```python
from build123d import *

# Parameters (mm, degrees)
SKETCH1_W           = 152.4
SKETCH1_H           = 101.6
BOSS_EXTRUDE1_DEPTH = 53.34
CUT_EXTRUDE1_START  = -12.7
SKETCH2_R           = 6.35
CUT_EXTRUDE1_DEPTH  = 127
FILLET2_R           = 2.54


with BuildPart() as part:
    # Sketch1 → Boss-Extrude1 (new body)
    with BuildSketch(Plane(origin=(0, 0, 0), x_dir=(1, 0, 0), z_dir=(0, 1, 0))):
        Rectangle(SKETCH1_W, SKETCH1_H)
    extrude(amount=-BOSS_EXTRUDE1_DEPTH)

    # Sketch2 → Cut-Extrude1 (cut)
    with BuildSketch(Plane(origin=(76.2, 0, 0), x_dir=(0, 0, -1), z_dir=(1, 0, 0)).offset(CUT_EXTRUDE1_START)):
        Circle(SKETCH2_R)
    extrude(amount=-CUT_EXTRUDE1_DEPTH, mode=Mode.SUBTRACT)

    # Fillet2
    fillet2_edges = [part.edges().sort_by_distance(p)[0] for p in [
        (63.5, -6.35, 0),
        (-63.5, -6.35, 0),
    ]]
    fillet(fillet2_edges, radius=FILLET2_R)


solid = part.part
```
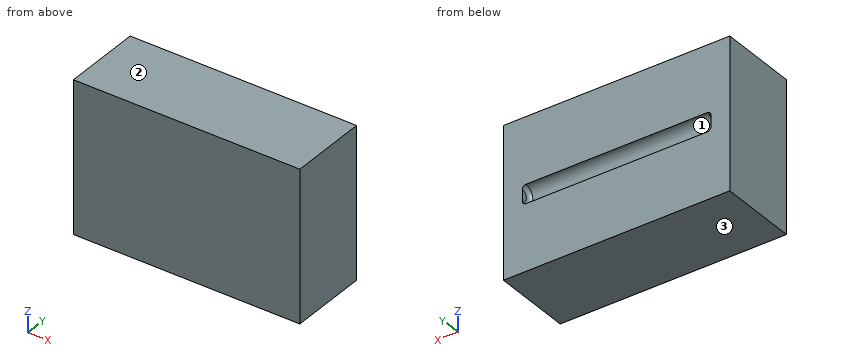
Read the model definition and answer for the solid it produces. Units are mm, in the model's axes. Face numbers are marked on the shaded views. Give positions to 0.01 mm unless a question says otherwise; leave off trailing zeros. Order: outer loops, then holes, each group sorted by start corner. A loop starts at its lowest first (then second) coordinate and runs counter-clockwise, first axis right, second up. Notation, with made-up numbers: (-4, -10.75) -> (10, -10.75) arc R23 ccw to (10, 12.25) -> close; hole circle Ø11 at (68.25, 71.25). An arc over 180 degrees is marked (long way). One line per item, written item: value. Start each with the question number.
(1) The part is cut by section A-A (z = 0). Determine the outline of the cut face in (x, y), and give its area (3 significant figures).
(2) Straight lines are drawn through the part: L1, parallel to Z at x = 60, y = -3; L2, parallel to Y at x = -59.5, z = -5. For each, find the intervals that lie inside material, in ascending order.
(3) For a pull along Z with two mould halves and no side action, classify the marked faces 1, 2 and 3 as released by +Z, released by -Z, zero draft, split by the parting line, or undercut.
Taken from the geometry:
1. outline: (-76.2, -53.34) -> (76.2, -53.34) -> (76.2, 0) -> (63.5, 0) -> (63.5, -3.81) arc R2.54 cw to (60.96, -6.35) -> (-60.96, -6.35) arc R2.54 cw to (-63.5, -3.81) -> (-63.5, 0) -> (-76.2, 0) -> close
1. area: 7,330 mm^2
2. L1: -50.8 to -5.6, 5.6 to 50.8
2. L2: -53.34 to -3.91
3. face 1: undercut
3. face 2: released by +Z
3. face 3: released by -Z
